Geometry: final body of the model. Coordinates: model frame, mm. A direction names the side the tool comes from. Coordinates: 2 decimals unless noted, no trailing zeros. Loops run counter-clockwise (first coordinate to the right, second up) from the corner with the lowest first, then second, coordinate; pieces in that order, holes last. Notation, with made-up numbers: (62.25, -33) - (72.25, -33) arc R34 cw to (72.25, 3) - close; hole circle Ø5 at (12, 12.5). An arc over 180 degrees is marked (long way). Answer in a Markdown table with one row per item.
from build123d import *

# Parameters (mm, degrees)
SKETCH1_R               = 4
SKETCH1_W               = 10
SKETCH1_H               = 30
BOSS_EXTRUDE1_DEPTH     = 8
SKETCH1_3_W             = 10
SKETCH1_3_H             = 30
BOSS_EXTRUDE2_DEPTH     = 40
FILLET1_R               = 3
CUT_EXTRUDE1_DEPTH      = 262.951140482
CUT_EXTRUDE1_DEPTH_BACK = 262.951140482
SKETCH2_R               = 5
SKETCH2_R_2             = 4
FILLET2_R               = 15
FILLET3_R               = 15


with BuildPart() as part:
    # Sketch1 → Boss-Extrude1 (new body)
    # profile 1 of 7: a face of its own
    with BuildSketch(Plane.XY):
        Polygon((-152.7, -38.1), (-114.3, -38.1), (114.3, -38.1), (114.3, 38.1), (114.3, 160.4), (-114.3, 160.4), (-152.7, 160.4), align=None)
        with Locations((-140, -25.4)):
            Circle(SKETCH1_R, mode=Mode.SUBTRACT)
        with Locations((-83.9, 0)):
            Rectangle(SKETCH1_W, SKETCH1_H, mode=Mode.SUBTRACT)
        with Locations((-53.9, 0)):
            Rectangle(SKETCH1_W, SKETCH1_H, mode=Mode.SUBTRACT)
        with Locations((101.6, -25.4)):
            Circle(SKETCH1_R, mode=Mode.SUBTRACT)
        with Locations((53.9, 0)):
            Rectangle(SKETCH1_W, SKETCH1_H, mode=Mode.SUBTRACT)
        with Locations((83.9, 0)):
            Rectangle(SKETCH1_W, SKETCH1_H, mode=Mode.SUBTRACT)
        with Locations((-135, 120)):
            Rectangle(SKETCH1_W, SKETCH1_H, mode=Mode.SUBTRACT)
        with Locations((-100, 120)):
            Rectangle(SKETCH1_W, SKETCH1_H, mode=Mode.SUBTRACT)
        with Locations((-140, 147.7)):
            Circle(SKETCH1_R, mode=Mode.SUBTRACT)
        with Locations((101.6, 147.7)):
            Circle(SKETCH1_R, mode=Mode.SUBTRACT)
    # profile 2 of 7: a face of its own
    with BuildSketch(Plane.XY):
        with Locations((-53.9, 0)):
            Rectangle(SKETCH1_W, SKETCH1_H)
    # profile 3 of 7: a face of its own
    with BuildSketch(Plane.XY):
        with Locations((-83.9, 0)):
            Rectangle(SKETCH1_W, SKETCH1_H)
    # profile 4 of 7: a face of its own
    with BuildSketch(Plane.XY):
        with Locations((53.9, 0)):
            Rectangle(SKETCH1_W, SKETCH1_H)
    # profile 5 of 7: a face of its own
    with BuildSketch(Plane.XY):
        with Locations((83.9, 0)):
            Rectangle(SKETCH1_W, SKETCH1_H)
    # profile 6 of 7: a face of its own
    with BuildSketch(Plane.XY):
        with Locations((-100, 120)):
            Rectangle(SKETCH1_W, SKETCH1_H)
    # profile 7 of 7: a face of its own
    with BuildSketch(Plane.XY):
        with Locations((-135, 120)):
            Rectangle(SKETCH1_W, SKETCH1_H)
    extrude(amount=BOSS_EXTRUDE1_DEPTH)

    # Sketch1<3> → Boss-Extrude2 (add)
    with BuildSketch(Plane.XY):
        with Locations((-83.9, 0)):
            Rectangle(SKETCH1_3_W, SKETCH1_3_H)
        with Locations((-53.9, 0)):
            Rectangle(SKETCH1_3_W, SKETCH1_3_H)
        with Locations((83.9, 0)):
            Rectangle(SKETCH1_3_W, SKETCH1_3_H)
        with Locations((53.9, 0)):
            Rectangle(SKETCH1_3_W, SKETCH1_3_H)
        with Locations((-100, 120)):
            Rectangle(SKETCH1_3_W, SKETCH1_3_H)
        with Locations((-135, 120)):
            Rectangle(SKETCH1_3_W, SKETCH1_3_H)
    extrude(amount=-BOSS_EXTRUDE2_DEPTH)

    # Fillet1
    fillet1_edges = [part.edges().sort_by_distance(p)[0] for p in [
        (-83.9, 15, 0),
        (-88.9, 0, 0),
        (-83.9, -15, 0),
        (-48.9, 0, 0),
        (-53.9, 15, 0),
        (-53.9, -15, 0),
        (88.9, 0, 0),
        (83.9, -15, 0),
        (83.9, 15, 0),
        (53.9, -15, 0),
        (53.9, 15, 0),
        (48.9, 0, 0),
    ]]
    fillet(fillet1_edges, radius=FILLET1_R)

    # Sketch2 → Cut-Extrude1 (cut, two sides: drawn at the far end of the back side and taken through both)
    with BuildSketch(Plane.ZY.offset(88.9).offset(-CUT_EXTRUDE1_DEPTH_BACK)):
        with Locations((-25, 0)):
            Circle(SKETCH2_R)
        with Locations((-25, 120)):
            Circle(SKETCH2_R_2)
    extrude(amount=CUT_EXTRUDE1_DEPTH + CUT_EXTRUDE1_DEPTH_BACK, mode=Mode.SUBTRACT)

    # Fillet2
    fillet2_edges = [part.edges().sort_by_distance(p)[0] for p in [
        (53.9, 15, -40),
        (53.9, -15, -40),
        (83.9, 15, -40),
        (83.9, -15, -40),
        (-53.9, 15, -40),
        (-53.9, -15, -40),
        (-83.9, -15, -40),
        (-83.9, 15, -40),
    ]]
    fillet(fillet2_edges, radius=FILLET2_R - 0.0001)  # a hair under: the kernel refuses the full size

    # Fillet3
    fillet3_edges = [part.edges().sort_by_distance(p)[0] for p in [
        (-135, 135, -40),
        (-135, 105, -40),
        (-100, 105, -40),
        (-100, 135, -40),
    ]]
    fillet(fillet3_edges, radius=FILLET3_R - 0.0001)  # a hair under: the kernel refuses the full size


solid = part.part
(1) First-contact query: pin 1 Ø8 at (x, z) = (85.5, -9.5) entering from +Y; pin 2 Ø15 at (y, z) = (-6.5, -12.5) entering from -X; pin 3 Ø9 at (y, z) = (0, -25) entering from +X; pin 4 Ø12 at (x, y) = (21.5, 107) entering from -Z. Flat tips, straight axial feed; report the tip coordinate or a pass-through.
Verdict:
| item | result |
|---|---|
| pin 1 | stops at y = 15 |
| pin 2 | stops at x = -88.9 |
| pin 3 | passes through |
| pin 4 | stops at z = 0 |
(2) Access query for faces 5 (the face through (-17, 160.4, 4)), 6 (the face through (-135, 105, -12)), 7 (the face through (58.9, -0.3, -19.7)), 8 (the face through (-100, 135, -12)). Directions: +Z, -Z, +X, -X, +Y, -Y. A direction counts if a zero-diameter tool reaches every point of the face in a straight line with its end or side. Return the directions, or none.
Verdict:
| item | result |
|---|---|
| face 5 | +Z, -Z, +X, -X, +Y |
| face 6 | -Z, +X, -X, -Y |
| face 7 | -Z, +Y, -Y |
| face 8 | -Z, +X, -X, +Y |
(3) Pull-direction query (Y, two-part tool) for faces 1 (the face through (103.446, 144.151, 3.944)), 2 (the face through (-84, 0, -30)), 3 (the face through (-152.7, 63, 4)), 4 (the face through (54, 15, -14)); classes: pulls with the +Y half, pulls with the -Y half, needs draft (parallel to the pull), parting line crosses it, or undercut.
Verdict:
| item | result |
|---|---|
| face 1 | undercut |
| face 2 | undercut |
| face 3 | needs draft |
| face 4 | pulls with the +Y half |
(4) Ray query, probe 1 along X at (y, z) = (-1, -31); probe 2 along X at (y, z) = (147, 2); probe 3 along Z at (x, y) = (-132, 120). Return the intervals inside material, ascending.
Verdict:
| item | result |
|---|---|
| probe 1 | x = -88.9 to -78.9, -58.9 to -48.9, 48.9 to 58.9, 78.9 to 88.9 |
| probe 2 | x = -152.7 to -143.94, -136.06 to 97.66, 105.54 to 114.3 |
| probe 3 | z = -40 to -29, -21 to 8 |
(5) Cut plane D-D on x = -67. Output: boundary loops of the cut face in (y, z).
Verdict:
| item | result |
|---|---|
| outline | (-38.1, 0) - (160.4, 0) - (160.4, 8) - (-38.1, 8) - close |
(6) Cut plane B-B on z = -11.5. Output: boundary loops of the cut face in (x, y), then the cut area to 3 significant figures.
Verdict:
| item | result |
|---|---|
| outline | (-140, 105) - (-130, 105) - (-130, 135) - (-140, 135) - close; (-105, 105) - (-95, 105) - (-95, 135) - (-105, 135) - close; (-88.9, -15) - (-78.9, -15) - (-78.9, 15) - (-88.9, 15) - close; (-58.9, -15) - (-48.9, -15) - (-48.9, 15) - (-58.9, 15) - close; (48.9, -15) - (58.9, -15) - (58.9, 15) - (48.9, 15) - close; (78.9, -15) - (88.9, -15) - (88.9, 15) - (78.9, 15) - close |
| area | 1,800 mm² |
(7) Cut plane A-A on x = 101.6. Output: boundary loops of the cut face in (y, z), then the cut area to 3 significant figures.
Verdict:
| item | result |
|---|---|
| outline | (-38.1, 0) - (-29.4, 0) - (-29.4, 8) - (-38.1, 8) - close; (-21.4, 0) - (143.7, 0) - (143.7, 8) - (-21.4, 8) - close; (151.7, 0) - (160.4, 0) - (160.4, 8) - (151.7, 8) - close |
| area | 1,460 mm² |
(8) Cut plane C-C on y = 147.7. Output: boundary loops of the cut face in (x, z).
Verdict:
| item | result |
|---|---|
| outline | (-152.7, 0) - (-144, 0) - (-144, 8) - (-152.7, 8) - close; (-136, 0) - (97.6, 0) - (97.6, 8) - (-136, 8) - close; (105.6, 0) - (114.3, 0) - (114.3, 8) - (105.6, 8) - close |
